from build123d import *

# Parameters (mm, degrees)
STOCK_OUTTER_CASE_1_START     = -75
STOCK_OUTTER_CASE_1_OUTLINE_W = 3
STOCK_OUTTER_CASE_1_OUTLINE_H = 184.8
STOCK_OUTTER_CASE_1_DEPTH     = 150
FILLET1_R                     = 0.2
BOSS_EXTRUDE1_DEPTH           = 29.8


# Read off the part's stored shape, not the designer's step: Stock-outter_case-1
with BuildPart() as part:
    # Stock-outter_case-1 outline → Stock-outter_case-1 (new body)
    with BuildSketch(Plane.XY.offset(STOCK_OUTTER_CASE_1_START)):
        with Locations((-154.5, 88.4)):
            Rectangle(STOCK_OUTTER_CASE_1_OUTLINE_W, STOCK_OUTTER_CASE_1_OUTLINE_H)
    extrude(amount=STOCK_OUTTER_CASE_1_DEPTH)

    # Fillet1
    fillet1_edges = [part.edges().sort_by_distance(p)[0] for p in [
        (-156, 180.8, 0),
        (-156, -4, 0),
        (-156, 88.4, 75),
        (-156, 88.4, -75),
    ]]
    fillet(fillet1_edges, radius=FILLET1_R)

    # Sketch1 → Boss-Extrude1 (add, symmetric)
    with BuildSketch(Plane(origin=(0, 74, 0), x_dir=(1, 0, 0), z_dir=(0, 1, 0))):
        with BuildLine():
            Line((-153, 75), (-151.139702343, 75))
            ThreePointArc((-151.139702343, 75), (-148.403541196, 75.482459034), (-145.997401465, 76.871644455))
            Line((-145.997401465, 76.871644455), (-143.384202565, 79.064378688))
            ThreePointArc((-143.384202565, 79.064378688), (-142.318796694, 79.204642032), (-141.741414955, 78.298334245))
            Line((-141.741414955, 78.298334245), (-141.741414955, 77.439817918))
            ThreePointArc((-141.741414955, 77.439817918), (-141.694568849, 77.228508787), (-141.56280876, 77.056795696))
            Line((-141.56280876, 77.056795696), (-139.290072737, 75.149743737))
            ThreePointArc((-139.290072737, 75.149743737), (-139.007347067, 74.606632777), (-139.191467271, 74.022678095))
            Line((-139.191467271, 74.022678095), (-139.448582314, 73.716260318))
            ThreePointArc((-139.448582314, 73.716260318), (-139.991693275, 73.433534647), (-140.575647957, 73.617654851))
            Line((-140.575647957, 73.617654851), (-143.026990175, 75.674575202))
            ThreePointArc((-143.026990175, 75.674575202), (-143.669777784, 75.908530759), (-144.312565394, 75.674575202))
            Line((-144.312565394, 75.674575202), (-146.663547874, 73.701866671))
            ThreePointArc((-146.663547874, 73.701866671), (-147.565850273, 73.180922138), (-148.591910703, 73))
            Line((-148.591910703, 73), (-150, 73))
            ThreePointArc((-150, 73), (-152.121320344, 72.121320344), (-153, 70))
            Line((-153, 70), (-153, 75))
        make_face()
    boss_extrude1 = extrude(amount=BOSS_EXTRUDE1_DEPTH, both=True)

    # Mirror1: Boss-Extrude1 across plane
    add(boss_extrude1.mirror(Plane.XY))


solid = part.part
Here's how the part is built. I have some questions about the finished solid (model axes, mm). A direction names the side the tool comes from. Round coordinates to 2 decimals unless told otherwise and drop trailing zeros. Write each loop counter-clockwise with the first axis right and the second up, starting at its lowest first coordinate (ties: lowest second). Pieces come first, ordered by that corner, then holes.
1. I need wall thicknesses on L1, parallel to X at y = 147, z = 50.5; L2, parallel to Z at x = -144, y = 73; L3, parallel to Z at x = -153.75, y = 99. Which ranges of each line are inside material? Lowest first, please.
2. Suppose I cut it at B-B (z = 29). List the corners of the cut face in (x, y) for me, and give its area (3 significant figures).
3. Will these pins go through, and if not, where does the flat tip stop? pin 1 Ø4.5 at (x, z) = (-146.5, -75.5) entering from -Y; pin 2 Ø12 at (y, z) = (18.5, 8) entering from +X; pin 3 Ø1.4 at (x, y) = (-154.5, 61.5) entering from +Z.
4. For faces 1 (the flat face through (-146, 44.2, -75)), 2 (the flat face through (-146, 103.8, 75)), 3 (the flat face through (-154, 90, 75)), which set-ups out of +Z, -Z, +X, -X, +Y, -Y let a thin tool reach every point of the face, with its end or its side?
5. Suppose I cut it at A-A (y = 168). List the corners of the cut face in (x, z) for me, and give its area (3 significant figures).
Answer sheet:
1. L1: x = -156 to -153
1. L2: z = -78.55 to -75.85, 75.85 to 78.55
1. L3: z = -75 to 75
2. outline: (-156, -3.8) arc R0.2 ccw to (-155.8, -4) - (-153, -4) - (-153, 180.8) - (-155.8, 180.8) arc R0.2 ccw to (-156, 180.6) - close
2. area: 554 mm2
3. pin 1: stops at y = 44.2
3. pin 2: stops at x = -153
3. pin 3: stops at z = 75
4. face 1: +Z, -Z, +X, -Y
4. face 2: +Z, -Z, +X, +Y
4. face 3: +Z, -X, +Y, -Y
5. outline: (-156, -74.8) arc R0.2 ccw to (-155.8, -75) - (-153, -75) - (-153, 75) - (-155.8, 75) arc R0.2 ccw to (-156, 74.8) - close
5. area: 450 mm2
